from build123d import *

# Parameters (mm, degrees)
SKETCH1_W           = 7.62
SKETCH1_H           = 25.4
SKETCH1_W_2         = 12.7
SKETCH1_H_2         = 12.7
BOSS_EXTRUDE1_DEPTH = 2.286
FILLET1_R           = 3.175


with BuildPart() as part:
    # Sketch1 → Boss-Extrude1 (new body)
    with BuildSketch(Plane.XY):
        with Locations((0, -19.05)):
            Rectangle(SKETCH1_W, SKETCH1_H)
        Rectangle(SKETCH1_W_2, SKETCH1_H_2)
    extrude(amount=BOSS_EXTRUDE1_DEPTH)

    # Fillet1
    # the kernel refuses this fillet: 3.175 mm, written as the material it adds along each edge
    with BuildSketch(Plane(origin=(-3.81, -6.35, 0), x_dir=(-1.0, -1.5648025307703881e-12, 0), z_dir=(0, 0, 1))) as fillet1_piece_1:
        with BuildLine():
            CenterArc((3.175, 3.110851973), FILLET1_R, 180, 78.463040967)
            Line((0, 3.110851973), (0, 0))
            Line((0, 0), (2.54, 0))
        make_face()
    extrude(amount=2.286)
    with BuildSketch(Plane(origin=(3.81, -6.35, 0), x_dir=(1.0, -1.5644528542271996e-12, 0), z_dir=(0, 0, 1))) as fillet1_piece_2:
        with BuildLine():
            CenterArc((3.175, -3.110851973), FILLET1_R, 101.536959033, 78.463040967)
            Line((0, -3.110851973), (0, 0))
            Line((0, 0), (2.54, 0))
        make_face()
    extrude(amount=2.286)
    # the kernel refuses this fillet: 3.175 mm, written as the material it takes off along each edge
    with BuildSketch(Plane(origin=(-3.81, -31.75, -7.9375), x_dir=(1, 0, 0), z_dir=(0, 0, 1)), Plane(origin=(3.81, -31.75, -7.9375), x_dir=(0, 1, 0), z_dir=(0, 0, 1))) as fillet1_2_piece_1:
        with BuildLine():
            CenterArc((FILLET1_R, FILLET1_R), FILLET1_R, 180, 90)
            Line((0, FILLET1_R), (0, 0))
            Line((0, 0), (FILLET1_R, 0))
        make_face()
    extrude(amount=18.161, mode=Mode.SUBTRACT)


solid = part.part
Verification items for the finished model (mm, model axes). A direction names the side the tool comes from. Coordinates: 2 decimals unless noted, no trailing zeros. Write each loop counter-clockwise with the first axis right and the second up, starting at its lowest first coordinate (ties: lowest second). Pieces come first, ordered by that corner, then holes. Notation, with made-up numbers: M 63.25,-34.5 L 81.25,-34.5 A20 ccw 81.25,-5.5 Z; hole C 37,67.5 d3. An arc over 180 degrees is marked long. Use CSV: the item, a comma, the result in double quotes.
Q1. Thickness scan on line 1 along X through (y, z) = (-23, 0.6); line 2 along Y through (x, z) = (-5.5, 1.5); line 3 along Y through (x, z) = (0.75, 1.3). Record the ranges inside material, lowest first. Write a range as [from, to].
Computed values:
line 1,"[-3.81, 3.81]"
line 2,"[-6.65, 6.35]"
line 3,"[-31.75, 6.35]"
Q2. Section check A-A, the plane z = 0.7. Enter the section's corners in (x, y) (3 decimals).
Computed values:
outline,"M -6.35,-6.35 A3.175 cw -3.81,-9.461 L -3.81,-28.575 A3.175 ccw -0.635,-31.75 L 0.635,-31.75 A3.175 ccw 3.81,-28.575 L 3.81,-9.461 A3.175 cw 6.35,-6.35 L 6.35,6.35 L -6.35,6.35 Z"
Q3. Section check C-C, the plane x = -3. Enter the section's corners in (y, z), and give its area (3 significant figures).
Computed values:
outline,"M -30.69,0 L 6.35,0 L 6.35,2.29 L -30.69,2.29 Z"
area,"84.7 mm²"
Q4. Section check B-B, the plane y = -13.5. Enter the section's corners in (x, z), and give its area (3 significant figures).
Computed values:
outline,"M -3.81,0 L 3.81,0 L 3.81,2.29 L -3.81,2.29 Z"
area,"17.4 mm²"
Q5. Go/stop test with a flat-tipped pin: P1, Ø0.7, axis at y = -21.5, z = 1, coming from the -X side. Record where the tip stops, or that it passes through.
Computed values:
P1,"x = -3.81"
Q6. Set-up check for faces 1 (the flat face through (0, 6.35, 1)), 2 (the flat face through (-3.81, -19, 1)), 3 (the flat face through (3.81, -19, 1)): record each of +Z, -Z, +X, -X, +Y, -Y from which the full face is reachable in a straight line by a thin tool's end or side.
Computed values:
face 1,"+Z, -Z, +X, -X, +Y"
face 2,"+Z, -Z, -X, -Y"
face 3,"+Z, -Z, +X, -Y"
